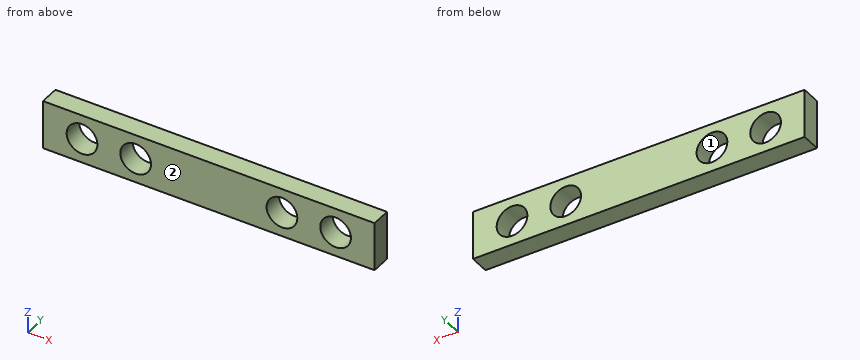
from build123d import *

# Parameters (mm, degrees)
SKETCH1_W           = 34
SKETCH1_H           = 5
BOSS_EXTRUDE2_DEPTH = 2
SKETCH4_R           = 1.575
CUT_EXTRUDE3_DEPTH  = 2
SKETCH5_R           = 1.575
CUT_EXTRUDE4_DEPTH  = 2


with BuildPart() as part:
    # Sketch1 → Boss-Extrude2 (new body)
    with BuildSketch(Plane(origin=(0, 0, 0), x_dir=(1, 0, 0), z_dir=(0, 1, 0))):
        Rectangle(SKETCH1_W, SKETCH1_H)
    extrude(amount=BOSS_EXTRUDE2_DEPTH)

    # Sketch4 → Cut-Extrude3 (cut)
    with BuildSketch(Plane(origin=(0, 2, 0), x_dir=(1, 0, 0), z_dir=(0, 1, 0))):
        with Locations((-13, 0)):
            Circle(SKETCH4_R)
        with Locations((13, 0)):
            Circle(SKETCH4_R)
    extrude(amount=-CUT_EXTRUDE3_DEPTH, mode=Mode.SUBTRACT)

    # Sketch5 → Cut-Extrude4 (cut)
    with BuildSketch(Plane(origin=(0, 2, 0), x_dir=(1, 0, 0), z_dir=(0, 1, 0))):
        with Locations((-7.5, 0)):
            Circle(SKETCH5_R)
        with Locations((7.5, 0)):
            Circle(SKETCH5_R)
    extrude(amount=-CUT_EXTRUDE4_DEPTH, mode=Mode.SUBTRACT)


solid = part.part
For this review, take the finished solid that the model builds, in its own axes (mm). Face numbers are marked on the shaded views. Round coordinates to 2 decimals unless told otherwise and drop trailing zeros. Order: outer loops, then holes, each group sorted by start corner. A loop starts at its lowest first (then second) coordinate and runs counter-clockwise, first axis right, second up. Notation, with made-up numbers: M -22.5,-35.75 L -5.5,-35.75 A20 cw -5.5,0.25 Z; hole C 50.25,-18 d7. An arc over 180 degrees is marked long. Use a Markdown table: item, result. Add a question column.
Item 1: To check wall thickness, follow line 1 along X through (y, z) = (1.55, 0) (3 decimals); line 2 along Z through (x, y) = (-13, 0.6) (3 decimals); line 3 along X through (y, z) = (0.65, 0.6). State the ranges of each line that lie inside material, in increasing order.
Item 2: Add section D-D, the plane x = 12.5. Give the boundary of the cut face in (y, z).
Item 3: Add section A-A, the plane z = 0. Give the boundary of the cut face in (x, y) (3 decimals), then the cut area to 3 significant figures.
Item 4: Insertion check: pin 1 (1.9 mm diameter, centred on x = 13, z = 0, fed in from +Y). The pin has a flat end and moves straight along its axis. Give the tip position at first contact, or say it passes through.
Item 5: Add section C-C, the plane y = 0.8. Give the boundary of the cut face in (x, z) (3 decimals), then the cut area to 3 significant figures.
Item 6: Mouldability with a two-part tool opening along X and no side actions: class the marked faces 1 and 2 as released by +X, released by -X, zero draft, split by the parting line, or undercut.
Item 7: Add section B-B, the plane x = -7.5. Give the boundary of the cut face in (y, z) (3 decimals).
Geometry results:
| question | item | result |
|---|---|---|
| 1 | line 1 | x = -17 to -14.575, -11.425 to -9.075, -5.925 to 5.925, 9.075 to 11.425, 14.575 to 17 |
| 1 | line 2 | z = -2.5 to -1.575, 1.575 to 2.5 |
| 1 | line 3 | x = -17 to -14.46, -11.54 to -8.96, -6.04 to 6.04, 8.96 to 11.54, 14.46 to 17 |
| 2 | outline | M 0,-2.5 L 2,-2.5 L 2,-1.49 L 0,-1.49 Z; M 0,1.49 L 2,1.49 L 2,2.5 L 0,2.5 Z |
| 3 | outline | M -17,0 L -14.575,0 L -14.575,2 L -17,2 Z; M -11.425,0 L -9.075,0 L -9.075,2 L -11.425,2 Z; M -5.925,0 L 5.925,0 L 5.925,2 L -5.925,2 Z; M 9.075,0 L 11.425,0 L 11.425,2 L 9.075,2 Z; M 14.575,0 L 17,0 L 17,2 L 14.575,2 Z |
| 3 | area | 42.8 mm² |
| 4 | pin 1 | passes through |
| 5 | outline | M -17,-2.5 L 17,-2.5 L 17,2.5 L -17,2.5 Z; hole C -13,0 d3.15; hole C -7.5,0 d3.15; hole C 7.5,0 d3.15; hole C 13,0 d3.15 |
| 5 | area | 139 mm² |
| 6 | face 1 | undercut |
| 6 | face 2 | zero draft |
| 7 | outline | M 0,-2.5 L 2,-2.5 L 2,-1.575 L 0,-1.575 Z; M 0,1.575 L 2,1.575 L 2,2.5 L 0,2.5 Z |
